Source: CAD feature listing. Evaluate the final solid. Frame: model axes, mm. Face numbers are marked on the shaded views. A direction names the side the tool comes from. Round coordinates to 2 decimals unless told otherwise and drop trailing zeros. Loops run counter-clockwise (first coordinate to the right, second up) from the corner with the lowest first, then second, coordinate; pieces in that order, holes last. Notation, with made-up numbers: (68, -27) - (91, -27) arc R20 ccw to (91, -9) - close; hole circle Ø9 at (31.5, 2). An arc over 180 degrees is marked (long way). One line per question, with ' | ' between items. Start each with the question number.
1. Ray query, line 1 (Z direction, x = 0, y = 2); line 2 (Z direction, x = 0, y = 0.7); line 3 (Y direction, x = 1, z = 5). Return the intervals inside material, ascending.
2. Mould query, pull axis Z, two halves, no side actions, for the marked faces 3, 4 and 5. Classes: pulls with the +Z half, pulls with the -Z half, needs draft (parallel to the pull), parting line crosses it, or undercut.
3. Cut plane D-D (z = 4). Return loops of the section in (x, y).
4. Access query for the marked faces 1 and 2. Directions: +Z, -Z, +X, -X, +Y, -Y. A direction counts if a zero-diameter tool reaches every point of the face in a straight line with its end or side. Return the directions, or none.
5. Cut plane C-C (z = 0). Return loops of the section in (x, y), then the cut area to 3 significant figures.
6. Cut plane B-B (y = 2.4). Return loops of the section in (x, z).
7. Cut plane A-A (x = 0). Return loops of the section in (y, z), then the cut area to 4 significant figures.
8. Pin query (flat end, axial travel): pin 1 (2.5 mm diameter, centred on x = 0, z = 0, fed in from +Y); pin 2 (1 mm diameter, centred on x = 1.5, y = 3, fed in from -Z); pin 3 (1 mm diameter, centred on x = 12, y = 0.5, fed in from -Z); pin 4 (2 mm diameter, centred on x = 11, z = 1.5, fed in from -Y). Return the tip coordinate at first contact, or that it passes through.
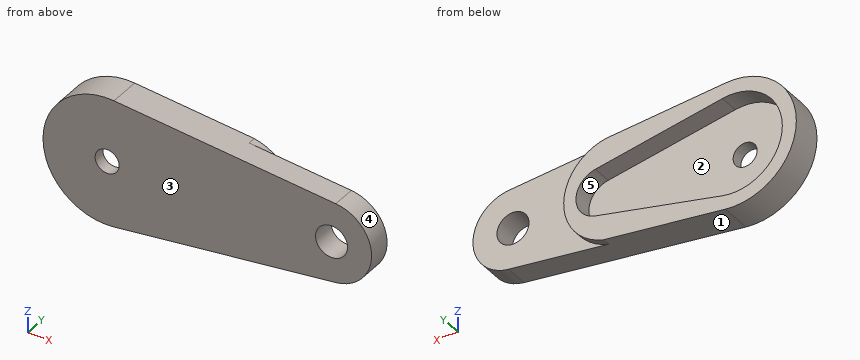
```python
from build123d import *

# Parameters (mm, degrees)
SKETCH1_R           = 1.5
SKETCH1_R_2         = 2
BOSS_EXTRUDE1_DEPTH = 4
CUT_EXTRUDE1_DEPTH  = 2.5
CUT_EXTRUDE2_START  = -1
SKETCH3_R           = 2
CUT_EXTRUDE2_DEPTH  = 1


with BuildPart() as part:
    # Sketch1 → Boss-Extrude1 (new body)
    with BuildSketch(Plane(origin=(0, 0, 0), x_dir=(1, 0, 0), z_dir=(0, 1, 0))):
        with BuildLine():
            Line((28.535714286, 4.971218181), (0.857142857, 7.95394909))
            ThreePointArc((0.857142857, 7.95394909), (-8, 0), (0.857142857, -7.95394909))
            Line((0.857142857, -7.95394909), (28.535714286, -4.971218181))
            ThreePointArc((28.535714286, -4.971218181), (33, 0), (28.535714286, 4.971218181))
        make_face()
        with Locations(Location((0, 0, 0), (0, 0, 270))):
            Circle(SKETCH1_R, mode=Mode.SUBTRACT)
        with Locations(Location((28, 0, 0), (0, 0, 270))):
            Circle(SKETCH1_R_2, mode=Mode.SUBTRACT)
    extrude(amount=BOSS_EXTRUDE1_DEPTH)

    # Sketch2 → Cut-Extrude1 (cut)
    with BuildSketch(Plane(origin=(0, 4, 0), x_dir=(1, 0, 0), z_dir=(0, 1, 0))):
        with BuildLine():
            Line((17.090909091, 2.941228731), (1.231060606, 6.127559856))
            ThreePointArc((1.231060606, 6.127559856), (-6.25, 0), (1.231060606, -6.127559856))
            Line((1.231060606, -6.127559856), (17.090909091, -2.941228731))
            ThreePointArc((17.090909091, -2.941228731), (19.5, 0), (17.090909091, 2.941228731))
        make_face()
    extrude(amount=-CUT_EXTRUDE1_DEPTH, mode=Mode.SUBTRACT)

    # Sketch3 → Cut-Extrude2 (cut)
    with BuildSketch(Plane(origin=(0, 4, 0), x_dir=(1, 0, 0), z_dir=(0, 1, 0)).offset(CUT_EXTRUDE2_START)):
        with BuildLine():
            Line((28.535714286, 4.971218181), (16.073296283, 6.314207991))
            ThreePointArc((16.073296283, 6.314207991), (21.027764344, -0.131247863), (15.785851253, -6.345183982))
            Line((15.785851253, -6.345183982), (28.535714286, -4.971218181))
            ThreePointArc((28.535714286, -4.971218181), (33, 0), (28.535714286, 4.971218181))
        make_face()
        with Locations(Location((28, 0, 0), (0, 0, 270))):
            Circle(SKETCH3_R, mode=Mode.SUBTRACT)
    extrude(amount=CUT_EXTRUDE2_DEPTH, mode=Mode.SUBTRACT)


solid = part.part
```
Answers follow:
1) line 1: z = -8 to -6.25, 6.25 to 8 | line 2: z = -8 to -1.5, 1.5 to 8 | line 3: y = 0 to 1.5
2) face 3: needs draft | face 4: parting line crosses it | face 5: undercut
3) outline: (-6.93, 0) - (31, 0) - (31, 3) - (19.64, 3) - (19.64, 4) - (11.82, 4) - (11.82, 1.5) - (-4.8, 1.5) - (-4.8, 4) - (-6.93, 4) - close
4) face 1: -Z, +X, +Y, -Y | face 2: +Y
5) outline: (-8, 0) - (-1.5, 0) - (-1.5, 1.5) - (-6.25, 1.5) - (-6.25, 4) - (-8, 4) - close; (1.5, 0) - (26, 0) - (26, 3) - (21.03, 3) - (21.03, 4) - (19.5, 4) - (19.5, 1.5) - (1.5, 1.5) - close; (30, 0) - (33, 0) - (33, 3) - (30, 3) - close | area: 71.2 mm2
6) outline: (0.86, -7.95) - (28.54, -4.97) arc R5 ccw to (28.54, 4.97) - (0.86, 7.95) arc R8 ccw (long way) to start; hole (1.23, -6.13) - (17.09, -2.94) arc R3 ccw to (17.09, 2.94) - (1.23, 6.13) arc R6.25 ccw (long way) to start; hole circle Ø4 at (28, 0)
7) outline: (0, -8) - (4, -8) - (4, -6.25) - (1.5, -6.25) - (1.5, -1.5) - (0, -1.5) - close; (0, 1.5) - (1.5, 1.5) - (1.5, 6.25) - (4, 6.25) - (4, 8) - (0, 8) - close | area: 28.25 mm2
8) pin 1: passes through | pin 2: stops at z = -7.94 | pin 3: stops at z = -6.81 | pin 4: stops at y = 0
